Here's how the part is built. I have some questions about the finished solid (model axes, mm). Face numbers are marked on the shaded views. A direction names the side the tool comes from. Round coordinates to 2 decimals unless told otherwise and drop trailing zeros. Order: outer loops, then holes, each group sorted by start corner. A loop starts at its lowest first (then second) coordinate and runs counter-clockwise, first axis right, second up. Notation, with made-up numbers: (1, 38.25) -> (31, 38.25) arc R32 cw to (31, 74.25) -> close; hole circle Ø11 at (56, 4.5). An arc over 180 degrees is marked (long way). One line per item, written item: value.
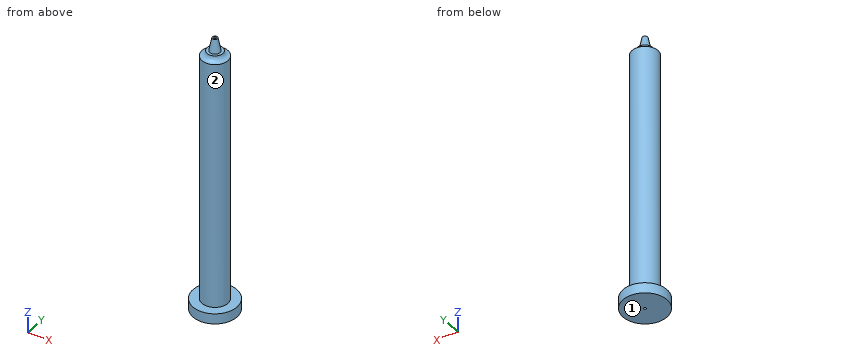
```python
from build123d import *

# Parameters (mm, degrees)
F0_R     = 8.5
F1_DEPTH = 4
F2_R     = 5
F3_DEPTH = 100
F8_R     = 0.5
F9_DEPTH = 129.4


with BuildPart() as f1:
    # F0 (on Top) → F1 (new body)
    with BuildSketch(Plane.XY):
        Circle(F0_R)
    extrude(amount=F1_DEPTH)

    # F2 (on Top) → F3 (join)
    with BuildSketch(Plane.XY):
        Circle(F2_R)
    extrude(amount=F3_DEPTH)

    # F4 (on Right) → F5 (revolve)
    with BuildSketch(Plane.YZ):
        with BuildLine():
            Line((3, 102), (0, 102))
            Line((0, 102), (0, 100))
            Line((0, 100), (5, 100))
            ThreePointArc((5, 100), (3.585786, 100.585786), (3, 102))
        make_face()
    revolve(axis=Axis((0, 0, 101), (0, 0, -1)))

    # F6 (on Right) → F7 (revolve)
    with BuildSketch(Plane.YZ):
        Polygon((0, 107), (0, 102), (2, 102), (1, 107), align=None)
    revolve(axis=Axis((0, 0, 104.5), (0, 0, 1)))

    # F8 (on face) → F9 (cut)
    with BuildSketch(Plane.XY.offset(107)):
        Circle(F8_R)
    extrude(amount=-F9_DEPTH, mode=Mode.SUBTRACT)


solid = f1.part
```
Q1. I need wall thicknesses on line 1 along Y through (x, z) = (0, 33.5); line 2 along Z through (x, y) = (2.5, 1.5); line 3 along Z through (x, y) = (2.5, -6.75). Which ranges of each line are inside material? Lowest first, please.
Answers:
line 1: -5 to -0.5, 0.5 to 5
line 2: 0 to 102
line 3: 0 to 4
Q2. Which directions (+Z, -Z, +X, -X, +Y, -Y) give clear straight access to the entire face, cutting with the end or side of a thin tool? Please do the marked faces 1 and 2.
Answers:
face 1: -Z, +X, -X, +Y, -Y
face 2: +Z
Q3. I want a section at B-B on y = -6. Write out the boundary of the cut face in (x, z), then the cut area to 3 significant figures.
Answers:
outline: (-6.02, 0) -> (6.02, 0) -> (6.02, 4) -> (-6.02, 4) -> close
area: 48.2 mm2
Q4. I want a section at C-C on x = 6.25. Write out the boundary of the cut face in (y, z), then the cut area to 3 significant figures.
Answers:
outline: (-5.76, 0) -> (5.76, 0) -> (5.76, 4) -> (-5.76, 4) -> close
area: 46.1 mm2
Q5. For P1, Ø3, axis at x = -4, y = 2.5, coming from the +Z side; P2, Ø5, axis at x = -1, z = 54, coming from the +Y side; P3, Ø4, axis at x = 6.5, z = 74, coming from the +Y side, each with a flat end and sliding along its axis, tell me the tip position at first contact or that it passes through.
Answers:
P1: z = 101.09
P2: y = 5
P3: y = 2.18
Q6. I want a section at A-A on z = 56.5. Write out the boundary of the cut face in (x, y).
Answers:
outline: circle Ø10 at (0, 0); hole circle Ø1 at (0, 0)
